Geometry: final body of the model. Coordinates: model frame, mm. A direction names the side the tool comes from. Round coordinates to 2 decimals unless told otherwise and drop trailing zeros. Loops run counter-clockwise (first coordinate to the right, second up) from the corner with the lowest first, then second, coordinate; pieces in that order, holes last. Notation, with made-up numbers: M 85.5,-15 L 124.5,-15 A10 ccw 124.5,-11 Z; hole C -15,67.5 d10. An arc over 180 degrees is marked long. Return JSON: item names as keys, results as strings.
from build123d import *

# Parameters (mm, degrees)
F0_W      = 14
F0_H      = 14
F1_DEPTH  = 8.2
F2_W      = 18
F2_H      = 7.2
F3_DEPTH  = 11.5
F5_DEPTH  = 14
F6_W      = 10.9
F6_H      = 7.2
F7_DEPTH  = 25
F8_W      = 15.1089467108
F8_H      = 7.5144236907
F9_DEPTH  = 8.2
F10_W     = 7.0144236907
F10_H     = 7.2
F11_DEPTH = 15.1
F12_W     = 1.5
F12_H     = 8.2
F13_DEPTH = 0.5


with BuildPart() as f1:
    # F0 (on Top) → F1 (new body)
    with BuildSketch(Plane.XY):
        Polygon((0, 11.4), (0, 0), (29.1, 0), (29.1, 11.4), (15.1, 11.4), align=None)
        with Locations((22.1, 18.4)):
            Rectangle(F0_W, F0_H)
    extrude(amount=F1_DEPTH)

    # F2 (on face) → F3 (cut)
    with BuildSketch(Plane.XZ):
        with Locations((20.1, 4.1)):
            Rectangle(F2_W, F2_H)
    extrude(amount=-F3_DEPTH, mode=Mode.SUBTRACT)

    # F4 (on face) → F5 (cut)
    with BuildSketch(Plane(origin=(0, 25.4, 0), x_dir=(-1, 0, 0), z_dir=(0, 1, 0))):
        with BuildLine():
            ThreePointArc((-17.5384761318, 0), (-16.3975752703, 1.8838162123), (-16, 4.05))
            ThreePointArc((-16, 4.05), (-16.4219059983, 6.2791811295), (-17.6292618059, 8.2))
            Line((-17.6292618059, 8.2), (-26.5707381941, 8.2))
            ThreePointArc((-26.5707381941, 8.2), (-28.1996261763, 4.1175315456), (-26.6615238682, 0))
            Line((-26.6615238682, 0), (-17.5384761318, 0))
        make_face()
    extrude(amount=-F5_DEPTH, mode=Mode.SUBTRACT)

    # F6 (on face) → F7 (cut)
    with BuildSketch(Plane(origin=(0, 0, 0), x_dir=(0, -1, 0), z_dir=(-1, 0, 0))):
        with Locations((-5.95, 4.1)):
            Rectangle(F6_W, F6_H)
    extrude(amount=-F7_DEPTH, mode=Mode.SUBTRACT)

    # F8 (on Top) → F9 (join)
    with BuildSketch(Plane.XY):
        with Locations((7.5544733554, 15.1720256545)):
            Rectangle(F8_W, F8_H)
    extrude(amount=F9_DEPTH)

    # F10 (on face) → F11 (cut)
    with BuildSketch(Plane(origin=(0, 0, 0), x_dir=(0, -1, 0), z_dir=(-1, 0, 0))):
        with Locations((-14.9220256545, 4.1)):
            Rectangle(F10_W, F10_H)
    extrude(amount=-F11_DEPTH, mode=Mode.SUBTRACT)

    # F12 (on face) → F13 (cut)
    with BuildSketch(Plane(origin=(0, 18.9292374998, 0), x_dir=(-1, 0, 0), z_dir=(0, 1, 0))):
        with Locations((-13.0113965198, 4.1)):
            Rectangle(F12_W, F12_H)
        with Locations((-6.8, 4.1)):
            Rectangle(F12_W, F12_H)
        with Locations((-9.8479721993, 4.1)):
            Rectangle(F12_W, F12_H)
        with Locations((-3.4783656076, 4.1)):
            Rectangle(F12_W, F12_H)
    extrude(amount=-F13_DEPTH, mode=Mode.SUBTRACT)


solid = f1.part
Q1. Section query C-C (y = 9). Output: boundary loops of the cut face in (x, z), plus the area to 3 significant figures.
Determined:
{"outline": "M 0,0 L 29.1,0 L 29.1,0.5 L 0,0.5 Z; M 0,7.7 L 29.1,7.7 L 29.1,8.2 L 0,8.2 Z", "area": "29.1 mm^2"}
Q2. Reachability of faces 5 (the flat face through (5, 0.5, 4)), 6 (the flat face through (7, 15, 0.5)), 7 (the flat face through (15.1, 22, 4)) from +Z, -Z, +X, -X, +Y, -Y: full face, straight path, thin tool, end or side. Return the list, or none.
Determined:
{"face 5": "+X, -X", "face 6": "-X", "face 7": "+Z, -Z, -X, +Y"}
Q3. Section query B-B (x = 2). Output: boundary loops of the cut face in (y, z), plus the area to 3 significant figures.
Determined:
{"outline": "M 0,0 L 11.4,0 L 11.4,0.5 L 0.5,0.5 L 0.5,7.7 L 11.4,7.7 L 11.4,8.2 L 0,8.2 Z; M 11.41,0 L 18.93,0 L 18.93,8.2 L 11.41,8.2 L 11.41,7.7 L 18.43,7.7 L 18.43,0.5 L 11.41,0.5 Z", "area": "26.1 mm^2"}
Q4. Pull-direction query (X, two-part tool) for faces 1 (the cylindrical face through (28.2, 18.5, 4.2)), 2 (the flat face through (29.1, 18, 4)), 3 (the flat face through (15.1, 15, 4)), 4 (the flat face through (14, 18.429, 4)); classes: pulls with the +X half, pulls with the -X half, needs draft (parallel to the pull), parting line crosses it, or undercut.
Determined:
{"face 1": "undercut", "face 2": "pulls with the +X half", "face 3": "pulls with the -X half", "face 4": "needs draft"}
Q5. Pin query (flat end, axial travel): pin 1 (1.5 mm diameter, centred on x = 21.5, z = 1.5, fed in from +Y); pin 2 (1.5 mm diameter, centred on x = 14, z = 2.5, fed in from +Y); pin 3 (1.7 mm diameter, centred on x = 28.5, z = 6, fed in from -Y); pin 4 (3 mm diameter, centred on y = 21.5, z = 4.5, fed in from -X). Return the tip coordinate at first contact, or that it passes through.
Determined:
{"pin 1": "passes through", "pin 2": "stops at y = 18.93", "pin 3": "stops at y = 11.5", "pin 4": "stops at x = 15.1"}
Q6. Material intervals for L1, parallel to Z at x = 6, y = 11; L2, parallel to X at y = 22.75, z = 3.75; L3, parallel to X at y = 18.75, z = 1.75, sorted ascending.
Determined:
{"L1": "z = 0 to 0.5, 7.7 to 8.2", "L2": "x = 15.1 to 16.01, 28.19 to 29.1", "L3": "x = 0 to 2.73, 4.23 to 6.05, 7.55 to 9.1, 10.6 to 12.26, 13.76 to 16.45, 27.75 to 29.1"}
Q7. Section query D-D (x = 13). Output: boundary loops of the cut face in (y, z), plus the area to 3 significant figures.
Determined:
{"outline": "M 0,0 L 11.4,0 L 11.4,0.5 L 0,0.5 Z; M 0,7.7 L 11.4,7.7 L 11.4,8.2 L 0,8.2 Z; M 11.41,0 L 18.43,0 L 18.43,0.5 L 11.41,0.5 Z; M 11.41,7.7 L 18.43,7.7 L 18.43,8.2 L 11.41,8.2 Z", "area": "18.4 mm^2"}
Q8. Section query A-A (z = 7.25). State how many separate pieces and enclosed holes the cut face has, plus the area to 3 significant figures.
Determined:
{"separate pieces": "7", "enclosed holes": "0", "area": "60.3 mm^2"}
